Work out the finished part from the listing and answer in its coordinate system (mm). Face numbers are marked on the shaded views. A direction names the side the tool comes from. Coordinates: 2 decimals unless noted, no trailing zeros. Order: outer loops, then holes, each group sorted by start corner. A loop starts at its lowest first (then second) coordinate and runs counter-clockwise, first axis right, second up.
```python
from build123d import *

# Parameters (mm, degrees)
BOSS_EXTRUDE1_DEPTH = 25
BOSS_EXTRUDE2_DEPTH = 20
BOSS_EXTRUDE3_DEPTH = 10


with BuildPart() as part:
    # Sketch1 → Boss-Extrude1 (new, symmetric)
    with BuildSketch(Plane.XY):
        with BuildLine():
            Line((-40, -27.5), (-40, 27.5))
            Line((-40, 27.5), (-20, 27.5))
            ThreePointArc((-20, 27.5), (-19.318516526, 32.676380902), (-17.320508076, 37.5))
            Line((-17.320508076, 37.5), (-8, 37.5))
            Line((-8, 37.5), (-8, 27.5))
            Line((-8, 27.5), (8, 27.5))
            Line((8, 27.5), (8, 37.5))
            Line((8, 37.5), (17.320508076, 37.5))
            ThreePointArc((17.320508076, 37.5), (19.318516526, 32.676380902), (20, 27.5))
            Line((20, 27.5), (40, 27.5))
            Line((40, 27.5), (40, -27.5))
            Line((40, -27.5), (29, -27.5))
            Line((29, -27.5), (29, 4.5))
            Line((29, 4.5), (-29, 4.5))
            Line((-29, 4.5), (-29, -27.5))
            Line((-29, -27.5), (-40, -27.5))
        make_face()
    extrude(amount=BOSS_EXTRUDE1_DEPTH, both=True)

    # Sketch2 → Boss-Extrude2 (add)
    with BuildSketch(Plane.XY.offset(25)):
        with BuildLine():
            Line((17.320508076, 37.5), (8, 37.5))
            Line((8, 37.5), (8, 27.5))
            Line((8, 27.5), (-8, 27.5))
            Line((-8, 27.5), (-8, 37.5))
            Line((-8, 37.5), (-17.320508076, 37.5))
            ThreePointArc((-17.320508076, 37.5), (0, 47.5), (17.320508076, 37.5))
        make_face()
    extrude(amount=-BOSS_EXTRUDE2_DEPTH)

    # Sketch3 → Boss-Extrude3 (add, symmetric)
    with BuildSketch(Plane.XY):
        Polygon((-40, 27.5), (-40, -27.5), (-58, -27.5), (-58, -7.5), (-40, 37.5), (-27, 37.5), (-27, 27.5), align=None)
        Polygon((27, 27.5), (40, 27.5), (40, -27.5), (58, -27.5), (58, -7.5), (40, 37.5), (27, 37.5), align=None)
    extrude(amount=BOSS_EXTRUDE3_DEPTH, both=True)


solid = part.part
```
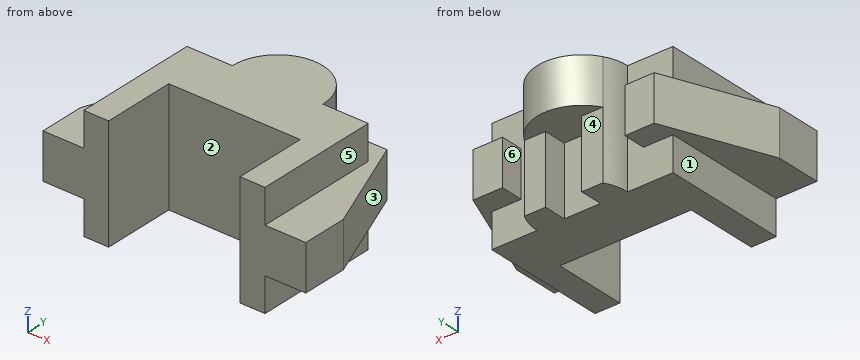
1. For the marked faces 4, 5 and 6, determine the directions among +Z, -Z, +X, -X, +Y, -Y from which every point of the face is accessible in a straight line to the end or side of a thin tool.
2. The part is cut by section C-C (x = -38.5). Determine the outline of the cut face in (y, z).
3. Consider probe 1 along X at (y, z) = (4, -20); probe 2 along X at (y, z) = (-20, 5); probe 3 along Z at (x, y) = (-12.5, 42.5). Determine where each line is inside the solid, lowest interval first.
4. Flat-ended cylindrical pins translate along their axes: pin 1 (7.5 mm diameter, centred on y = -12.5, z = -16.5, fed in from +X); pin 2 (10.5 mm diameter, centred on x = 12, z = -4, fed in from +Y); pin 3 (6 mm diameter, centred on x = 2, z = -5.5, fed in from -Y). Find the tip coordinate at first contact, or state that the pin passes through.
5. The mould has two halves that part along X. Classify the marked faces 1, 2 and 3: released by +X, released by -X, zero draft, split by the parting line, or undercut.
6. The part is cut by section A-A (y = -4). Determine the outline of the cut face in (x, z), plus the area to 3 significant figures.
7. The part is cut by section B-B (z = 20). Determine the outline of the cut face in (x, y), plus the area to 3 significant figures.
8. The part is cut by section D-D (y = -12). Determine the outline of the cut face in (x, z), plus the area to 3 significant figures.
Worked out:
1. face 4: -Z, +X, -X, +Y
1. face 5: +Z, +X, +Y, -Y
1. face 6: +Z, -Z, +Y
2. outline: (-27.5, -25) - (27.5, -25) - (27.5, -10) - (37.5, -10) - (37.5, 10) - (27.5, 10) - (27.5, 25) - (-27.5, 25) - close
3. probe 1: x = -40 to -29, 29 to 40
3. probe 2: x = -58 to -29, 29 to 58
3. probe 3: z = 5 to 25
4. pin 1: stops at x = 40
4. pin 2: stops at y = 37.5
4. pin 3: stops at y = 4.5
5. face 1: released by -X
5. face 2: undercut
5. face 3: released by +X
6. outline: (-56.6, -10) - (-40, -10) - (-40, -25) - (-29, -25) - (-29, 25) - (-40, 25) - (-40, 10) - (-56.6, 10) - close; (29, -25) - (40, -25) - (40, -10) - (56.6, -10) - (56.6, 10) - (40, 10) - (40, 25) - (29, 25) - close
6. area: 1,760 mm2
7. outline: (-40, -27.5) - (-29, -27.5) - (-29, 4.5) - (29, 4.5) - (29, -27.5) - (40, -27.5) - (40, 27.5) - (20, 27.5) arc R20 ccw to (-20, 27.5) - (-40, 27.5) - close
7. area: 3,170 mm2
8. outline: (-58, -10) - (-40, -10) - (-40, -25) - (-29, -25) - (-29, 25) - (-40, 25) - (-40, 10) - (-58, 10) - close; (29, -25) - (40, -25) - (40, -10) - (58, -10) - (58, 10) - (40, 10) - (40, 25) - (29, 25) - close
8. area: 1,820 mm2
